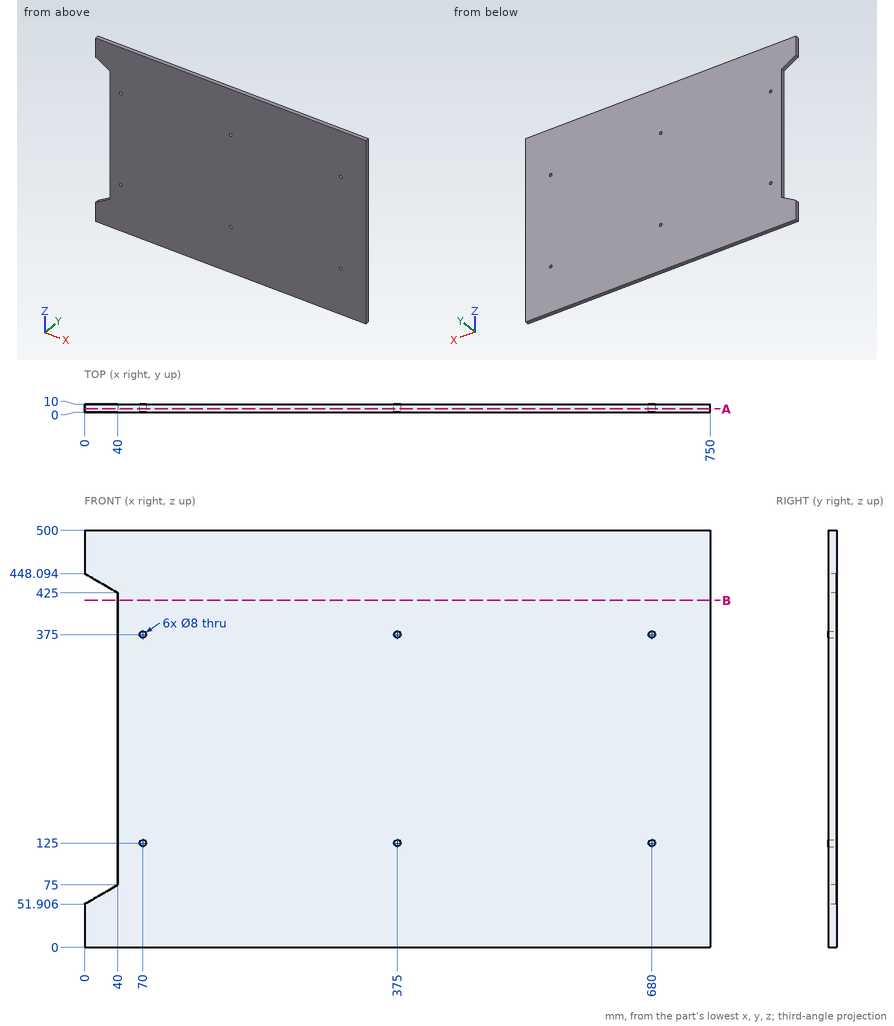
Study the drawing (mm; zero at the part's minimum x, y, z) and answer. Coordinates: 2 decimals unless noted, no trailing zeros. Write each loop counter-clockwise with the first axis right and the second up, starting at its lowest first coordinate (ties: lowest second). Pieces come first, ordered by that corner, then holes. Notation, with made-up numbers: (72.5, 73) - (86.5, 73) arc R20 cw to (86.5, 108) - close; hole circle Ø4 at (-20.75, 23.25). An arc over 180 degrees is marked (long way). Answer as a JSON object with one key per item and string values. Group by question number.
1. Consider L1, parallel to X at y = 5.25, z = 375; L2, parallel to Z at x = 375, y = 3; L3, parallel to X at y = 5.25, z = 365.5. Determine where each line is inside the solid, lowest interval first. Write a range as [from, to].
2. A cutting plane is placed at A-A (y = 4.25). Determine the outline of the cut face in (x, z).
3. Each of these flat-tipped pins is pushed along its axis until it touches: P1, Ø10.5, axis at x = 375, z = 375, coming from the +Y side; P2, Ø5, axis at y = 4.5, z = 266.5, coming from the -X side. Where does it stop, or does it pass through?
4. A cutting plane is placed at B-B (z = 416). Determine the outline of the cut face in (x, y), plus the area to 3 significant figures.
Worked out:
{
 "1": {"L1": "x = [40, 66], [74, 371], [379, 676], [684, 750]", "L2": "z = [0, 121], [129, 371], [379, 500]", "L3": "x = [40, 750]"},
 "2": {"outline": "(0, 0) - (750, 0) - (750, 500) - (0, 500) - (0, 448.09) - (40, 425) - (40, 75) - (0, 51.91) - close; hole circle Ø8 at (70, 125); hole circle Ø8 at (70, 375); hole circle Ø8 at (375, 125); hole circle Ø8 at (375, 375); hole circle Ø8 at (680, 125); hole circle Ø8 at (680, 375)"},
 "3": {"P1": "stops at y = 10", "P2": "stops at x = 40"},
 "4": {"outline": "(40, 0) - (750, 0) - (750, 10) - (40, 10) - close", "area": "7,100 mm²"}
}
